Source: CAD feature listing. Evaluate the final solid. Frame: model axes, mm. Round coordinates to 2 decimals unless told otherwise and drop trailing zeros. Write each loop counter-clockwise with the first axis right and the second up, starting at its lowest first coordinate (ties: lowest second). Pieces come first, ordered by that corner, then holes. Notation, with made-up numbers: M 89,40.5 L 130,40.5 A12 ccw 130,60.5 Z; hole C -25,-0.5 d2. An arc over 180 degrees is marked long. Put each result on its own line as item: value. Start each with the question number.
```python
from build123d import *

# Parameters (mm, degrees)
F1_DEPTH = 101.6
F4_R     = 3.175
F5_DEPTH = 101.601


with BuildPart() as f1:
    # F0 (on Right) → F1 (new body)
    with BuildSketch(Plane.YZ):
        Polygon((3.6661742094, 6.35), (-3.6661742094, 6.35), (-7.3323484187, 0), (-3.6661742094, -6.35), (3.6661742094, -6.35), (7.3323484187, 0), align=None)
    extrude(amount=F1_DEPTH)

    # F2 (on Top) → F3 (revolve, cut)
    with BuildSketch(Plane.XY):
        Polygon((100.0125, 6.35), (101.6, 6.35), (101.6, 7.3323484187), (99.0219, 7.3323484187), (99.0219, 5.9436), (100.0125, 5.9436), align=None)
    revolve(axis=Axis((50.8, 0, 0), (1, 0, 0)), mode=Mode.SUBTRACT)

    # F4 (on face) → F5 (cut, through all)
    with BuildSketch(Plane.YZ.offset(101.6)):
        Circle(F4_R)
    extrude(amount=-F5_DEPTH, mode=Mode.SUBTRACT)


solid = f1.part
```
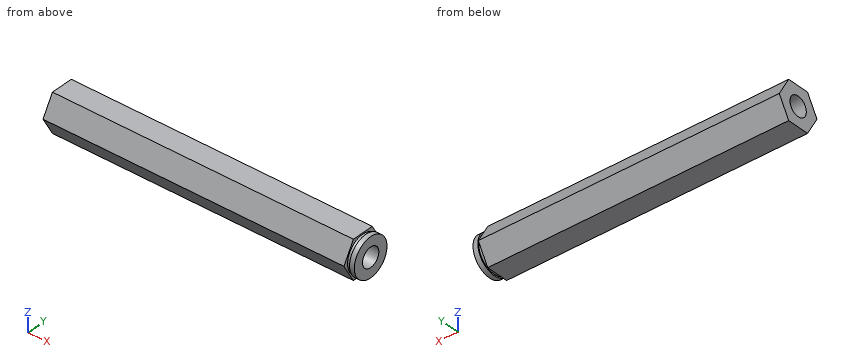
(1) Section query C-C (z = 2). Return loops of the section in (x, y), and give its area (3 significant figures).
(2) Section query D-D (y = -5). Return loops of the section in (x, z).
(3) Ray query, line 1 along Z through (x, y) = (73.5, 0) (3 decimals); line 2 along Z through (x, y) = (91, 0.5); line 3 along Y through (x, z) = (88, 1.25). Return the intervals inside material, ascending.
(4) Contact query for a flat-ended pin moving along its axis: P1, Ø1.5, axis at x = 84.5, z = -1, coming from the +Y side. Output: stop coordinate, or through.
(5) Section query B-B (x = 9). Return loops of the section in (y, z) (3 decimals), and give its area (3 significant figures).
Entries:
1. outline: M 0,-6.18 L 99.02,-6.18 L 99.02,-5.6 L 100.01,-5.6 L 100.01,-6.03 L 101.6,-6.03 L 101.6,-2.47 L 0,-2.47 Z; M 0,2.47 L 101.6,2.47 L 101.6,6.03 L 100.01,6.03 L 100.01,5.6 L 99.02,5.6 L 99.02,6.18 L 0,6.18 Z
1. area: 753 mm2
2. outline: M 0,-4.04 L 99.02,-4.04 L 99.02,-3.21 L 100.01,-3.21 L 100.01,-3.91 L 101.6,-3.91 L 101.6,3.91 L 100.01,3.91 L 100.01,3.21 L 99.02,3.21 L 99.02,4.04 L 0,4.04 Z
3. line 1: -6.35 to -3.175, 3.175 to 6.35
3. line 2: -6.35 to -3.14, 3.14 to 6.35
3. line 3: -6.61 to -2.92, 2.92 to 6.61
4. P1: y = 7.19
5. outline: M -7.332,0 L -3.666,-6.35 L 3.666,-6.35 L 7.332,0 L 3.666,6.35 L -3.666,6.35 Z; hole C 0,0 d6.35
5. area: 108 mm2
